The model under review builds one solid part; all positions refer to its coordinate system, in mm. A direction names the side the tool comes from. Round coordinates to 2 decimals unless told otherwise and drop trailing zeros. Write each loop counter-clockwise with the first axis right and the second up, starting at its lowest first coordinate (ties: lowest second). Pieces come first, ordered by that corner, then holes. Notation, with made-up numbers: M 51,37.5 L 96,37.5 A29 cw 96,57.5 Z; hole C 0,40.25 d11. An arc over 180 degrees is marked long. One line per item, written item: value. Start each with the question number.
1) Wall thickness on probe 1 along X at (y, z) = (-23.5, -82.5); probe 2 along X at (y, z) = (-1, 0); probe 3 along Z at (x, y) = (24, -9.5): over which ranges is each line inside the solid? List them lowest first.
2) Take a section at B-B, the plane z = 0. Write out the cut boundary in (x, y), and give its area (3 significant figures).
3) Take a section at D-D, the plane x = 34.5. Write out the cut boundary in (y, z).
4) For P1, Ø6.5, axis at x = -0.5, z = -88, coming from the -Y side; P2, Ø8, axis at x = 2.5, z = 45, coming from the +Y side, all flat-tipped, find the tip position at first contact; note any pin that passes through.
5) Mouldability with a two-part tool opening along Z and no side actions: class faces 1 (the face through (0, -20, -87)), 2 (the face through (-1, -15, 92.5)), 3 (the face through (86, -25, 22.5)) as +Z half, -Z half, draft (parallel to the pull), parting line (faces both ways), or undercut.
6) Take a section at A-A, the plane y = -27. Write out the cut boundary in (x, z), and give its area (3 significant figures).
7) Take a section at C-C, the plane y = -13.75. Write out the cut boundary in (x, z).
8) Tool access review of faces 4 (the face through (65, -30, 66)), 5 (the face through (-86, -25, -22.5)), 6 (the face through (-24.78, -16.2, 78.69)), 7 (the face through (-22.5, -25, -86)): name each direction out of +Z, -Z, +X, -X, +Y, -Y from which nothing blocks a thin tool from reaching the whole face with its end or side.
from build123d import *

# Parameters (mm, degrees)
BOSS_EXTRUDE1_START = -30
SKETCH2_W           = 185
SKETCH2_H           = 185
SKETCH2_R           = 85.5
SKETCH2_R_2         = 3
BOSS_EXTRUDE1_DEPTH = 30
SKETCH3_W           = 45
SKETCH3_H           = 10
CUT_EXTRUDE1_DEPTH  = 210.000598085
SKETCH4_W           = 45
SKETCH4_H           = 10
CUT_EXTRUDE2_DEPTH  = 210.000598085


with BuildPart() as part:
    # Sketch1 → Revolve1 (revolve)
    with BuildSketch(Plane.XY, mode=Mode.PRIVATE) as revolve1_sk:
        Polygon((53, -2), (82.5, -2), (82.5, -30), (85.5, -30), (85.5, 0), (53, 0), align=None)
    revolve(revolve1_sk.sketch.rotate(Axis((0, 0, 0), (0, -1, 0)), 90), axis=Axis((0, 0, 0), (0, -1, 0)))

    # Sketch2 → Boss-Extrude1 (add)
    with BuildSketch(Plane.XZ.offset(30).offset(BOSS_EXTRUDE1_START)):
        Rectangle(SKETCH2_W, SKETCH2_H)
        Circle(SKETCH2_R, mode=Mode.SUBTRACT)
        with Locations(Location((-82.5, -82.5, 0), (0, 0, 270))):
            Circle(SKETCH2_R_2, mode=Mode.SUBTRACT)
        with Locations(Location((82.5, -82.5, 0), (0, 0, 270))):
            Circle(SKETCH2_R_2, mode=Mode.SUBTRACT)
        with Locations(Location((82.5, 82.5, 0), (0, 0, 270))):
            Circle(SKETCH2_R_2, mode=Mode.SUBTRACT)
        with Locations(Location((-82.5, 82.5, 0), (0, 0, 270))):
            Circle(SKETCH2_R_2, mode=Mode.SUBTRACT)
    extrude(amount=BOSS_EXTRUDE1_DEPTH)

    # Sketch3 → Cut-Extrude1 (cut, through all)
    with BuildSketch(Plane.ZY.offset(92.5)):
        with Locations((0, -25)):
            Rectangle(SKETCH3_W, SKETCH3_H)
    extrude(amount=-CUT_EXTRUDE1_DEPTH, mode=Mode.SUBTRACT)

    # Sketch4 → Cut-Extrude2 (cut, through all)
    with BuildSketch(Plane(origin=(0, 0, -92.5), x_dir=(-1, 0, 0), z_dir=(0, 0, -1))):
        with Locations((0, -25)):
            Rectangle(SKETCH4_W, SKETCH4_H)
    extrude(amount=-CUT_EXTRUDE2_DEPTH, mode=Mode.SUBTRACT)


solid = part.part
Checked values:
1. probe 1: x = -92.5 to -85.5, -79.5 to -22.5, 22.5 to 79.5, 85.5 to 92.5
1. probe 2: x = -92.5 to -53, 53 to 92.5
1. probe 3: z = -92.5 to -78.93, 78.93 to 92.5
2. outline: M -92.5,-20 L -82.5,-20 L -82.5,-2 L -53,-2 L -53,0 L -92.5,0 Z; M 53,-2 L 82.5,-2 L 82.5,-20 L 92.5,-20 L 92.5,0 L 53,0 Z
2. area: 518 mm2
3. outline: M -30,-92.5 L 0,-92.5 L 0,-40.23 L -2,-40.23 L -2,-74.94 L -30,-74.94 Z; M -30,74.94 L -2,74.94 L -2,40.23 L 0,40.23 L 0,92.5 L -30,92.5 Z
4. P1: stops at y = -20
4. P2: passes through
5. face 1: draft
5. face 2: +Z half
5. face 3: undercut
6. outline: M -92.5,-92.5 L -22.5,-92.5 L -22.5,-79.37 A82.5 cw -79.37,-22.5 L -92.5,-22.5 Z; M -92.5,22.5 L -79.37,22.5 A82.5 cw -22.5,79.37 L -22.5,92.5 L -92.5,92.5 Z; M 22.5,-92.5 L 92.5,-92.5 L 92.5,-22.5 L 79.37,-22.5 A82.5 cw 22.5,-79.37 Z; M 22.5,79.37 A82.5 cw 79.37,22.5 L 92.5,22.5 L 92.5,92.5 L 22.5,92.5 Z; hole C -82.5,-82.5 d6; hole C -82.5,82.5 d6; hole C 82.5,-82.5 d6; hole C 82.5,82.5 d6
6. area: 10,700 mm2
7. outline: M -92.5,-92.5 L 92.5,-92.5 L 92.5,92.5 L -92.5,92.5 Z; hole C -82.5,-82.5 d6; hole C -82.5,82.5 d6; hole C 0,0 d165; hole C 82.5,-82.5 d6; hole C 82.5,82.5 d6
8. face 4: +Z, -Z, +X, -X, -Y
8. face 5: +X, -X, -Y
8. face 6: -Y
8. face 7: +Z, -Z, -Y
